Geometry check sheet. Reference: the model listing, model coordinates, mm. Face numbers are marked on the shaded views. Round coordinates to 2 decimals unless told otherwise and drop trailing zeros. Order: outer loops, then holes, each group sorted by start corner. A loop starts at its lowest first (then second) coordinate and runs counter-clockwise, first axis right, second up. Notation, with made-up numbers: (20.25, -29) -> (54.25, -29) arc R22 cw to (54.25, -19) -> close; hole circle Ø4 at (85, 28). An arc over 180 degrees is marked (long way). Use a Markdown table: item, result. Add a question column.
Item 1: Sectioned sample at B-B, the plane y = 1.1. State how many separate pieces and enclosed holes the cut face has, and give its area (3 significant figures).
Item 2: Gauge pin test, flat end, axial feed: pin 1 Ø13 at (x, z) = (-122.8, 23.246) entering from +Y. Record the tip position at first contact, or that the pin passes through.
Item 3: Sectioned sample at A-A, the plane x = -122.8. Record the cut outline in (y, z).
Item 4: Mould release check, pull along Y, two halves, no side actions. Record for the marked faces 1 and 2: pulls with the +Y half, pulls with the -Y half, needs draft (parallel to the pull), parting line crosses it, or undercut.
Item 5: Material ranges on probe 1 along Z at (x, y) = (-63.5, 1.5); probe 2 along X at (y, z) = (1.3, 18); probe 3 along Z at (x, y) = (142.5, 0.7), recorded low to high. Write a range as [from, to].
from build123d import *

# Parameters (mm, degrees)
SKETCH1_R           = 10.8
SKETCH1_R_2         = 1.5
BOSS_EXTRUDE1_DEPTH = 2


with BuildPart() as part:
    # Sketch1 → Boss-Extrude1 (new body)
    with BuildSketch(Plane(origin=(0, 0, 0), x_dir=(1, 0, 0), z_dir=(0, 1, 0))):
        with BuildLine():
            Line((-165.1, 63.246), (165.1, 63.246))
            ThreePointArc((165.1, 63.246), (174.080256121, 59.526256121), (177.8, 50.546))
            Line((177.8, 50.546), (177.8, -50.546))
            ThreePointArc((177.8, -50.546), (174.080256121, -59.526256121), (165.1, -63.246))
            Line((165.1, -63.246), (-165.1, -63.246))
            ThreePointArc((-165.1, -63.246), (-174.080256121, -59.526256121), (-177.8, -50.546))
            Line((-177.8, -50.546), (-177.8, 50.546))
            ThreePointArc((-177.8, 50.546), (-174.080256121, 59.526256121), (-165.1, 63.246))
        make_face()
        with Locations((-122.8, -23.246)):
            Circle(SKETCH1_R, mode=Mode.SUBTRACT)
        with Locations((107.99, 0)):
            Circle(SKETCH1_R_2, mode=Mode.SUBTRACT)
        with Locations((147.8, 0)):
            Circle(SKETCH1_R_2, mode=Mode.SUBTRACT)
        with BuildLine():
            Line((-118.893595003, 34.346), (-126.706404997, 34.346))
            ThreePointArc((-126.706404997, 34.346), (-128.848729166, 33.973704171), (-130.739847555, 32.900471545))
            ThreePointArc((-130.739847555, 32.900471545), (-135.3, 23.246), (-130.739847555, 13.591528455))
            ThreePointArc((-130.739847555, 13.591528455), (-128.848729166, 12.518295829), (-126.706404997, 12.146))
            Line((-126.706404997, 12.146), (-118.893595003, 12.146))
            ThreePointArc((-118.893595003, 12.146), (-116.751270834, 12.518295829), (-114.860152445, 13.591528455))
            ThreePointArc((-114.860152445, 13.591528455), (-110.3, 23.246), (-114.860152445, 32.900471545))
            ThreePointArc((-114.860152445, 32.900471545), (-116.751270834, 33.973704171), (-118.893595003, 34.346))
        make_face(mode=Mode.SUBTRACT)
        with BuildLine():
            Line((-70.115, 31.014285463), (-70.115, 28.985714537))
            ThreePointArc((-70.115, 28.985714537), (-69.600932797, 26.482838513), (-68.141964286, 24.385205474))
            ThreePointArc((-68.141964286, 24.385205474), (-62.8, 22.25), (-57.458035714, 24.385205474))
            ThreePointArc((-57.458035714, 24.385205474), (-55.999067203, 26.482838513), (-55.485, 28.985714537))
            Line((-55.485, 28.985714537), (-55.485, 31.014285463))
            ThreePointArc((-55.485, 31.014285463), (-55.999067203, 33.517161487), (-57.458035714, 35.614794526))
            ThreePointArc((-57.458035714, 35.614794526), (-62.8, 37.75), (-68.141964286, 35.614794526))
            ThreePointArc((-68.141964286, 35.614794526), (-69.600932797, 33.517161487), (-70.115, 31.014285463))
        make_face(mode=Mode.SUBTRACT)
        with BuildLine():
            Line((-40.115, 31.014285463), (-40.115, 28.985714537))
            ThreePointArc((-40.115, 28.985714537), (-39.600932797, 26.482838513), (-38.141964286, 24.385205474))
            ThreePointArc((-38.141964286, 24.385205474), (-32.8, 22.25), (-27.458035714, 24.385205474))
            ThreePointArc((-27.458035714, 24.385205474), (-25.999067203, 26.482838513), (-25.485, 28.985714537))
            Line((-25.485, 28.985714537), (-25.485, 31.014285463))
            ThreePointArc((-25.485, 31.014285463), (-25.999067203, 33.517161487), (-27.458035714, 35.614794526))
            ThreePointArc((-27.458035714, 35.614794526), (-32.8, 37.75), (-38.141964286, 35.614794526))
            ThreePointArc((-38.141964286, 35.614794526), (-39.600932797, 33.517161487), (-40.115, 31.014285463))
        make_face(mode=Mode.SUBTRACT)
        with BuildLine():
            Line((-70.115, 1.014285463), (-70.115, -1.014285463))
            ThreePointArc((-70.115, -1.014285463), (-69.600932797, -3.517161487), (-68.141964286, -5.614794526))
            ThreePointArc((-68.141964286, -5.614794526), (-62.8, -7.75), (-57.458035714, -5.614794526))
            ThreePointArc((-57.458035714, -5.614794526), (-55.999067203, -3.517161487), (-55.485, -1.014285463))
            Line((-55.485, -1.014285463), (-55.485, 1.014285463))
            ThreePointArc((-55.485, 1.014285463), (-55.999067203, 3.517161487), (-57.458035714, 5.614794526))
            ThreePointArc((-57.458035714, 5.614794526), (-62.8, 7.75), (-68.141964286, 5.614794526))
            ThreePointArc((-68.141964286, 5.614794526), (-69.600932797, 3.517161487), (-70.115, 1.014285463))
        make_face(mode=Mode.SUBTRACT)
        with BuildLine():
            Line((-70.115, -28.985714537), (-70.115, -31.014285463))
            ThreePointArc((-70.115, -31.014285463), (-69.600932797, -33.517161487), (-68.141964286, -35.614794526))
            ThreePointArc((-68.141964286, -35.614794526), (-62.8, -37.75), (-57.458035714, -35.614794526))
            ThreePointArc((-57.458035714, -35.614794526), (-55.999067203, -33.517161487), (-55.485, -31.014285463))
            Line((-55.485, -31.014285463), (-55.485, -28.985714537))
            ThreePointArc((-55.485, -28.985714537), (-55.999067203, -26.482838513), (-57.458035714, -24.385205474))
            ThreePointArc((-57.458035714, -24.385205474), (-62.8, -22.25), (-68.141964286, -24.385205474))
            ThreePointArc((-68.141964286, -24.385205474), (-69.600932797, -26.482838513), (-70.115, -28.985714537))
        make_face(mode=Mode.SUBTRACT)
        with BuildLine():
            Line((-40.115, -28.985714537), (-40.115, -31.014285463))
            ThreePointArc((-40.115, -31.014285463), (-39.600932797, -33.517161487), (-38.141964286, -35.614794526))
            ThreePointArc((-38.141964286, -35.614794526), (-32.8, -37.75), (-27.458035714, -35.614794526))
            ThreePointArc((-27.458035714, -35.614794526), (-25.999067203, -33.517161487), (-25.485, -31.014285463))
            Line((-25.485, -31.014285463), (-25.485, -28.985714537))
            ThreePointArc((-25.485, -28.985714537), (-25.999067203, -26.482838513), (-27.458035714, -24.385205474))
            ThreePointArc((-27.458035714, -24.385205474), (-32.8, -22.25), (-38.141964286, -24.385205474))
            ThreePointArc((-38.141964286, -24.385205474), (-39.600932797, -26.482838513), (-40.115, -28.985714537))
        make_face(mode=Mode.SUBTRACT)
        with BuildLine():
            Line((-25.485, 1.014285463), (-25.485, -1.014285463))
            ThreePointArc((-25.485, -1.014285463), (-25.999067203, -3.517161487), (-27.458035714, -5.614794526))
            ThreePointArc((-27.458035714, -5.614794526), (-32.8, -7.75), (-38.141964286, -5.614794526))
            ThreePointArc((-38.141964286, -5.614794526), (-39.600932797, -3.517161487), (-40.115, -1.014285463))
            Line((-40.115, -1.014285463), (-40.115, 1.014285463))
            ThreePointArc((-40.115, 1.014285463), (-39.600932797, 3.517161487), (-38.141964286, 5.614794526))
            ThreePointArc((-38.141964286, 5.614794526), (-32.8, 7.75), (-27.458035714, 5.614794526))
            ThreePointArc((-27.458035714, 5.614794526), (-25.999067203, 3.517161487), (-25.485, 1.014285463))
        make_face(mode=Mode.SUBTRACT)
        with BuildLine():
            Line((-1.63, 1.61592079), (-1.63, -1.61592079))
            ThreePointArc((-1.63, -1.61592079), (-1.367126425, -3.424066772), (-0.60027027, -5.08250762))
            ThreePointArc((-0.60027027, -5.08250762), (7.2, -9.31), (15.00027027, -5.08250762))
            ThreePointArc((15.00027027, -5.08250762), (15.767126425, -3.424066772), (16.03, -1.61592079))
            Line((16.03, -1.61592079), (16.03, 1.61592079))
            ThreePointArc((16.03, 1.61592079), (15.767126425, 3.424066772), (15.00027027, 5.08250762))
            ThreePointArc((15.00027027, 5.08250762), (7.2, 9.31), (-0.60027027, 5.08250762))
            ThreePointArc((-0.60027027, 5.08250762), (-1.367126425, 3.424066772), (-1.63, 1.61592079))
        make_face(mode=Mode.SUBTRACT)
        with BuildLine():
            Line((125.321896428, 23.415), (130.468103572, 23.415))
            ThreePointArc((130.468103572, 23.415), (132.18640119, 23.651903134), (133.776487756, 24.34493597))
            ThreePointArc((133.776487756, 24.34493597), (141.575, 23.415), (142.50493597, 15.616487756))
            ThreePointArc((142.50493597, 15.616487756), (141.811903134, 14.02640119), (141.575, 12.308103572))
            Line((141.575, 12.308103572), (141.575, -12.308103572))
            ThreePointArc((141.575, -12.308103572), (141.811903134, -14.02640119), (142.50493597, -15.616487756))
            ThreePointArc((142.50493597, -15.616487756), (141.575, -23.415), (133.776487756, -24.34493597))
            ThreePointArc((133.776487756, -24.34493597), (132.18640119, -23.651903134), (130.468103572, -23.415))
            Line((130.468103572, -23.415), (125.321896428, -23.415))
            ThreePointArc((125.321896428, -23.415), (123.60359881, -23.651903134), (122.013512244, -24.34493597))
            ThreePointArc((122.013512244, -24.34493597), (114.215, -23.415), (113.28506403, -15.616487756))
            ThreePointArc((113.28506403, -15.616487756), (113.978096866, -14.02640119), (114.215, -12.308103572))
            Line((114.215, -12.308103572), (114.215, 12.308103572))
            ThreePointArc((114.215, 12.308103572), (113.978096866, 14.02640119), (113.28506403, 15.616487756))
            ThreePointArc((113.28506403, 15.616487756), (114.215, 23.415), (122.013512244, 24.34493597))
            ThreePointArc((122.013512244, 24.34493597), (123.60359881, 23.651903134), (125.321896428, 23.415))
        make_face(mode=Mode.SUBTRACT)
    extrude(amount=BOSS_EXTRUDE1_DEPTH)


solid = part.part
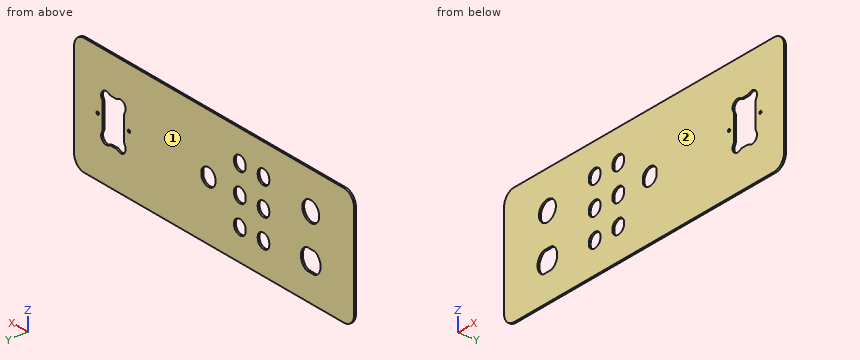
Found:
| question | item | result |
|---|---|---|
| 1 | separate pieces | 1 |
| 1 | enclosed holes | 12 |
| 1 | area | 41,200 mm2 |
| 2 | pin 1 | passes through |
| 3 | outline | (0, -63.25) -> (2, -63.25) -> (2, -34.35) -> (0, -34.35) -> close; (0, -12.15) -> (2, -12.15) -> (2, 12.45) -> (0, 12.45) -> close; (0, 34.05) -> (2, 34.05) -> (2, 63.25) -> (0, 63.25) -> close |
| 4 | face 1 | pulls with the +Y half |
| 4 | face 2 | pulls with the -Y half |
| 5 | probe 1 | z = [-63.25, -37.72], [-22.28, -7.72], [7.72, 22.28], [37.72, 63.25] |
| 5 | probe 2 | x = [-177.8, -132.24], [-113.36, 112.42], [143.37, 177.8] |
| 5 | probe 3 | z = [-63.25, -22.24], [-15.61, 15.61], [22.24, 63.25] |
